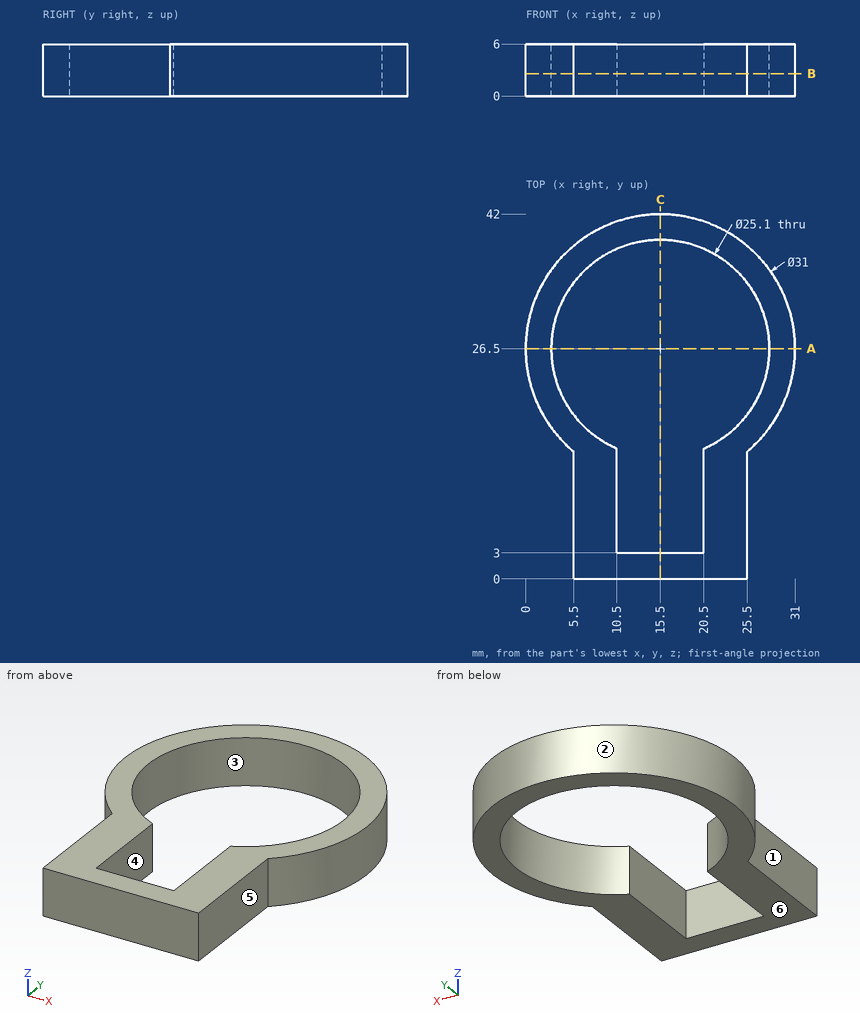
Verification items for this drawing (mm, ordinates from the low corner). A direction names the side the tool comes from. Give positions to 0.01 mm unless a question says otherwise; leave off trailing zeros. Loops run counter-clockwise (first coordinate to the right, second up) from the corner with the lowest first, then second, coordinate; pieces in that order, holes last.
(1) Section check B-B on z = 2.6. Record the cut outline in (x, y).
From the geometry:
outline: (5.5, 0) - (25.5, 0) - (25.5, 14.66) arc R15.5 ccw (long way) to (5.5, 14.66) - close; hole (10.5, 3) - (20.5, 3) - (20.5, 14.99) arc R12.55 ccw (long way) to (10.5, 14.99) - close
(2) Thickness scan on L1, parallel to X at y = 26.5, z = 4.35; L2, parallel to Y at x = 15.5, z = 3.1; L3, parallel to X at y = 4, z = 1.8. Record the ranges inside material, lowest first.
From the geometry:
L1: x = 0 to 2.95, 28.05 to 31
L2: y = 0 to 3, 39.05 to 42
L3: x = 5.5 to 10.5, 20.5 to 25.5
(3) Depth check by flat-ended pin: pin 1 Ø1 at (y, z) = (33.5, 3) entering from -X; pin 2 Ø1 at (y, z) = (19.5, 1) entering from +X; pin 3 Ø3 at (y, z) = (7.5, 4.5) entering from +X. Enter the tip coordinate at first touch or a pass-through.
From the geometry:
pin 1: stops at x = 1.43
pin 2: stops at x = 29.57
pin 3: stops at x = 25.5
(4) Release check for a two-part mould opening along Y. For the marked faces 1, 2 and 3 record: released by +Y, released by -Y, zero draft, split by the parting line, or undercut.
From the geometry:
face 1: zero draft
face 2: split by the parting line
face 3: undercut
(5) Set-up check for the marked faces 4, 5 and 6: record each of +Z, -Z, +X, -X, +Y, -Y from which the full face is reachable in a straight line by a thin tool's end or side.
From the geometry:
face 4: +Z, -Z
face 5: +Z, -Z, +X, -Y
face 6: -Z, +X, -X, +Y, -Y
(6) Section check C-C on x = 15.5. Record the cut outline in (y, z).
From the geometry:
outline: (0, 0) - (3, 0) - (3, 6) - (0, 6) - close; (39.05, 0) - (42, 0) - (42, 6) - (39.05, 6) - close
(7) Section check A-A on y = 26.5. Record the cut outline in (x, z), then the cut area to 3 significant figures.
From the geometry:
outline: (0, 0) - (2.95, 0) - (2.95, 6) - (0, 6) - close; (28.05, 0) - (31, 0) - (31, 6) - (28.05, 6) - close
area: 35.4 mm2
